Input: dimensioned drawing with shaded views. Units: mm. Origin: part minimum x, y, z. Coordinates: 2 decimals unless noted, no trailing zeros. Loops run counter-clockwise (first coordinate to the right, second up) from the corner with the lowest first, then second, coordinate; pieces in that order, holes last.
Item 1: Section B-B on y = 13.75. Return loops of the section in (x, z) (1 decimal), and give its area (3 significant figures).
Item 2: Section A-A on x = 28.5. Return loops of the section in (y, z), and give its area (3 significant figures).
Item 3: Ray query, line 1 along X through (y, z) = (1.9, 12.25) (1 decimal); line 2 along X through (y, z) = (5.75, 16.5). Return the intervals inside material, ascending.
Item 4: Contact query for flat-ended pins moving along their axis: P1, Ø1.8, axis at x = 12.25, z = 12.25, coming from the -Y side (1 decimal); P2, Ø2, axis at x = 44.5, y = 12.5, coming from the -Z side; P3, Ø2.5, axis at x = 44.75, z = 44.75, coming from the +Y side; P4, Ø3.5, axis at x = 44.75, z = 12.25, coming from the -Y side. Output: stop coordinate, or through.
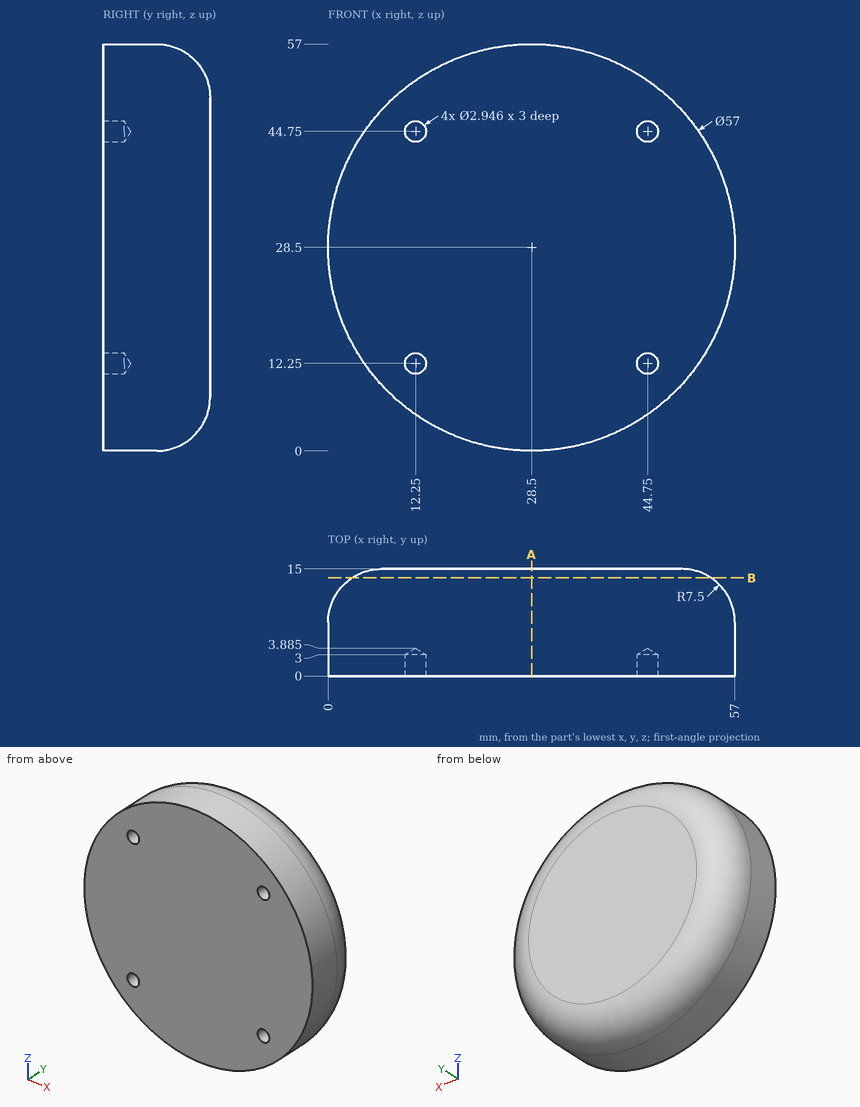
Results found:
1. outline: circle Ø50.3 at (28.5, 28.5)
1. area: 1,990 mm2
2. outline: (0, 0) - (7.5, 0) arc R7.5 ccw to (15, 7.5) - (15, 49.5) arc R7.5 ccw to (7.5, 57) - (0, 57) - close
2. area: 831 mm2
3. line 1: x = 5.1 to 10.8, 13.7 to 43.3, 46.2 to 51.9
3. line 2: x = 2.65 to 54.35
4. P1: stops at y = 3.3
4. P2: stops at z = 6.06
4. P3: stops at y = 14.96
4. P4: stops at y = 0
